The listing builds one solid part. Answer for the finished solid, in the listing's coordinates (mm). Face numbers are marked on the shaded views. A direction names the side the tool comes from. Give positions to 0.01 mm unless a question says otherwise; leave off trailing zeros. Loops run counter-clockwise (first coordinate to the right, second up) from the corner with the lowest first, then second, coordinate; pieces in that order, holes last. Notation, with made-up numbers: (74, 71) - (114, 71) arc R29 ccw to (114, 98) - close; hole circle Ø3 at (69, -36). An arc over 180 degrees is marked (long way). Write each question's results on one line, items separated by ' | '.
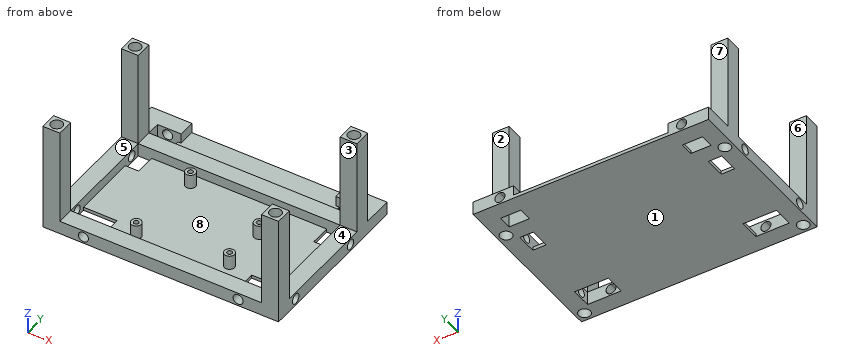
from build123d import *

# Parameters (mm, degrees)
F0_W      = 10
F0_H      = 10
F1_DEPTH  = 60
F3_W      = 10
F3_H      = 8
F3_W_2    = 120
F3_H_2    = 63
F3_H_3    = 10
F3_W_3    = 14
F4_DEPTH  = 8
F6_DEPTH  = 2
F7_R      = 3
F7_R_2    = 1.5
F8_DEPTH  = 10.5
F9_R      = 3.5
F10_DEPTH = 75
F11_R     = 3
F12_DEPTH = 10
F13_R     = 3
F14_DEPTH = 10
F16_DEPTH = 10
F18_DEPTH = 10


with BuildPart() as f1:
    # F0 (on Top) → F1 (new body)
    with BuildSketch(Plane.XY):
        with Locations((-65, 28)):
            Rectangle(F0_W, F0_H)
        with Locations((65, 28)):
            Rectangle(F0_W, F0_H)
        with Locations((-65, -45)):
            Rectangle(F0_W, F0_H)
        with Locations((65, -45)):
            Rectangle(F0_W, F0_H)
    extrude(amount=-F1_DEPTH)

    # F3 (on offset) → F4 (join)
    with BuildSketch(Plane.XY.offset(-65)):
        with Locations((-65, 37)):
            Rectangle(F3_W, F3_H)
        Polygon((-60, 33), (-70, 33), (-70, 23), (-70, -40), (-70, -50), (-60, -50), (60, -50), (70, -50), (70, -40), (70, 23), (70, 33), (60, 33), align=None)
        with Locations((0, -8.5)):
            Rectangle(F3_W_2, F3_H_2, mode=Mode.SUBTRACT)
        with Locations((-65, 46)):
            Rectangle(F3_W, F3_H_3)
        with Locations((65, 37)):
            Rectangle(F3_W, F3_H)
        with Locations((-53, 46)):
            Rectangle(F3_W_3, F3_H_3)
        with Locations((53, 46)):
            Rectangle(F3_W_3, F3_H_3)
        with Locations((65, 46)):
            Rectangle(F3_W, F3_H_3)
    extrude(amount=F4_DEPTH)

    # F5 (on offset) → F6 (join)
    with BuildSketch(Plane.XY.offset(-65)):
        Polygon((-48, 33), (-52, 33), (-52, 11), (-60, 11), (-60, -28), (-40, -28), (-40, -40), (40, -40), (40, -28), (60, -28), (60, 11), (52, 11), (52, 33), (48, 33), (48, 41), (46, 41), (46, 51), (-46, 51), (-46, 41), (-48, 41), align=None)
    extrude(amount=F6_DEPTH)

    # F7 (on offset) → F8 (join)
    with BuildSketch(Plane.XY.offset(-65)):
        with Locations((-24.34509, 15.832442)):
            Circle(F7_R)
        with Locations((-24.34509, 15.832442)):
            Circle(F7_R_2, mode=Mode.SUBTRACT)
        with Locations((26.337272, 0.330886)):
            Circle(F7_R)
        with Locations((26.337272, 0.330886)):
            Circle(F7_R_2, mode=Mode.SUBTRACT)
        with Locations((26.613058, -27.667755)):
            Circle(F7_R)
        with Locations((26.613058, -27.667755)):
            Circle(F7_R_2, mode=Mode.SUBTRACT)
        with Locations((-25.65, -32.65)):
            Circle(F7_R)
        with Locations((-25.65, -32.65)):
            Circle(F7_R_2, mode=Mode.SUBTRACT)
    extrude(amount=F8_DEPTH)

    # F9 (on Top) → F10 (cut)
    with BuildSketch(Plane.XY):
        with Locations((-65, 28)):
            Circle(F9_R)
        with Locations((-65, -45)):
            Circle(F9_R)
        with Locations((65, -45)):
            Circle(F9_R)
        with Locations((65, 28)):
            Circle(F9_R)
    extrude(amount=-F10_DEPTH, mode=Mode.SUBTRACT)

    # F11 (on face) → F12 (cut)
    with BuildSketch(Plane.YZ.offset(70)):
        with Locations((-34, -61)):
            Circle(F11_R)
        with Locations((17, -61)):
            Circle(F11_R)
    extrude(amount=-F12_DEPTH, mode=Mode.SUBTRACT)

    # F13 (on face) → F14 (cut)
    with BuildSketch(Plane(origin=(-70, 0, 0), x_dir=(0, -1, 0), z_dir=(-1, 0, 0))):
        with Locations((-17, -61)):
            Circle(F13_R)
        with Locations((34, -61)):
            Circle(F13_R)
    extrude(amount=-F14_DEPTH, mode=Mode.SUBTRACT)

    # F15 (on face) → F16 (cut)
    with BuildSketch(Plane.XZ.offset(50)):
        with BuildLine():
            ThreePointArc((-46, -58), (-48.12132, -63.12132), (-43, -61))
            ThreePointArc((-43, -61), (-43.87868, -58.87868), (-46, -58))
        make_face()
        with BuildLine():
            ThreePointArc((46, -58), (43.87868, -63.12132), (49, -61))
            ThreePointArc((49, -61), (48.12132, -58.87868), (46, -58))
        make_face()
    extrude(amount=-F16_DEPTH, mode=Mode.SUBTRACT)

    # F17 (on face) → F18 (cut)
    with BuildSketch(Plane(origin=(0, 51, 0), x_dir=(-1, 0, 0), z_dir=(0, 1, 0))):
        with BuildLine():
            ThreePointArc((-54, -58), (-56.12132, -63.12132), (-51, -61))
            ThreePointArc((-51, -61), (-51.87868, -58.87868), (-54, -58))
        make_face()
        with BuildLine():
            ThreePointArc((54, -58), (51.87868, -63.12132), (57, -61))
            ThreePointArc((57, -61), (56.12132, -58.87868), (54, -58))
        make_face()
    extrude(amount=-F18_DEPTH, mode=Mode.SUBTRACT)


solid = f1.part
Item 1: A cutting plane is placed at D-D, the plane x = 35. Determine the outline of the cut face in (y, z).
Values found:
outline: (-50, -65) - (51, -65) - (51, -63) - (33, -63) - (33, -57) - (23, -57) - (23, -63) - (-40, -63) - (-40, -57) - (-50, -57) - close
Item 2: For a pull along Y with two mould halves and no side action, classify the marked faces 1, 2 and 3 as released by +Y, released by -Y, zero draft, split by the parting line, or undercut.
Values found:
face 1: zero draft | face 2: released by +Y | face 3: undercut
Item 3: A cutting plane is placed at B-B, the plane z = -17. Determine the outline of the cut face in (x, y), plus the area to 3 significant figures.
Values found:
outline: (-70, -50) - (-60, -50) - (-60, -40) - (-70, -40) - close; (-70, 23) - (-60, 23) - (-60, 33) - (-70, 33) - close; (60, -50) - (70, -50) - (70, -40) - (60, -40) - close; (60, 23) - (70, 23) - (70, 33) - (60, 33) - close; hole circle Ø7 at (-65, -45); hole circle Ø7 at (-65, 28); hole circle Ø7 at (65, -45); hole circle Ø7 at (65, 28) | area: 246 mm²
Item 4: A cutting plane is placed at C-C, the plane y = 36. Determine the outline of the cut face in (x, z), plus the area to 3 significant figures.
Values found:
outline: (-70, -65) - (-60, -65) - (-60, -57) - (-70, -57) - close; (-48, -65) - (48, -65) - (48, -63) - (-48, -63) - close; (60, -65) - (70, -65) - (70, -57) - (60, -57) - close | area: 352 mm²
Item 5: Find the intervals of material crossed by line 1 along Y through (x, z) = (65, -33); line 2 along Y through (x, z) = (-38, -59); line 3 along X through (y, z) = (5, -60), in increasing order. Write a range as [from, to].
Values found:
line 1: y = [-50, -48.5], [-41.5, -40], [23, 24.5], [31.5, 33] | line 2: y = [-50, -40], [23, 33] | line 3: x = [-70, -60], [60, 70]
Item 6: Flat-ended cylindrical pins translate along their axes: P1, Ø3, axis at x = 62.5, z = -38, coming from the +Y side; P2, Ø5, axis at x = -15.5, y = 26, coming from the +Z side; P3, Ø5, axis at y = -36.5, z = -13.5, coming from the -X side; P4, Ø5, axis at y = 17, z = -61, coming from the -X side. Find the tip coordinate at first contact, or state that the pin passes through.
Values found:
P1: stops at y = 33 | P2: stops at z = -57 | P3: passes through | P4: stops at x = -52
Item 7: A cutting plane is placed at A-A, the plane y = -45. Determine the outline of the cut face in (x, z), plus the area to 3 significant figures.
Values found:
outline: (-70, -65) - (-68.5, -65) - (-68.5, 0) - (-70, 0) - close; (-61.5, -65) - (61.5, -65) - (61.5, 0) - (60, 0) - (60, -57) - (-60, -57) - (-60, 0) - (-61.5, 0) - close; (68.5, -65) - (70, -65) - (70, 0) - (68.5, 0) - close; hole (-46, -58) arc R3 ccw (long way) to (-43, -61) arc R3 ccw to start; hole (46, -58) arc R3 ccw (long way) to (49, -61) arc R3 ccw to start | area: 1,290 mm²
Item 8: For the marked faces 4, 5, 6, 7 and 8, determine the directions among +Z, -Z, +X, -X, +Y, -Y from which every point of the face is accessible in a straight line to the end or side of a thin tool.
Values found:
face 4: +Z, +X | face 5: +Z, -X | face 6: +Z, +X, -X | face 7: +Z, +X, -X, +Y | face 8: +Z
